from build123d import *

# Parameters (mm, degrees)
F1_DEPTH = 76.2
F2_R     = 46.767549
F3_DEPTH = 50.8


with BuildPart() as f1:
    # F0 (on Right) → F1 (new body)
    with BuildSketch(Plane.YZ):
        with BuildLine():
            ThreePointArc((-47.755212, -55.394912), (-16.585087, -35.145607), (-4.485609, 0))
            ThreePointArc((-4.485609, 0), (-16.585087, 35.145607), (-47.755212, 55.394912))
            ThreePointArc((-47.755212, 55.394912), (-118.673271, 0), (-47.755212, -55.394912))
        make_face()
        with BuildLine():
            ThreePointArc((-47.755212, 55.394912), (-16.585087, 35.145607), (-4.485609, 0))
            ThreePointArc((-4.485609, 0), (-16.585087, -35.145607), (-47.755212, -55.394912))
            Line((-47.755212, -55.394912), (75.465698, -24.644182))
            ThreePointArc((75.465698, -24.644182), (43.915552, 0), (75.465698, 24.644182))
            Line((75.465698, 24.644182), (-47.755212, 55.394912))
        make_face()
        with BuildLine():
            ThreePointArc((94.715552, 0), (89.332716, 15.635637), (75.465698, 24.644182))
            ThreePointArc((75.465698, 24.644182), (43.915552, 0), (75.465698, -24.644182))
            ThreePointArc((75.465698, -24.644182), (89.332716, -15.635637), (94.715552, 0))
        make_face()
    extrude(amount=F1_DEPTH)

    # F2 (on face) → F3 (cut)
    with BuildSketch(Plane.YZ.offset(76.2)):
        with Locations((-61.57944, 0)):
            Circle(F2_R)
    extrude(amount=-F3_DEPTH, mode=Mode.SUBTRACT)


solid = f1.part
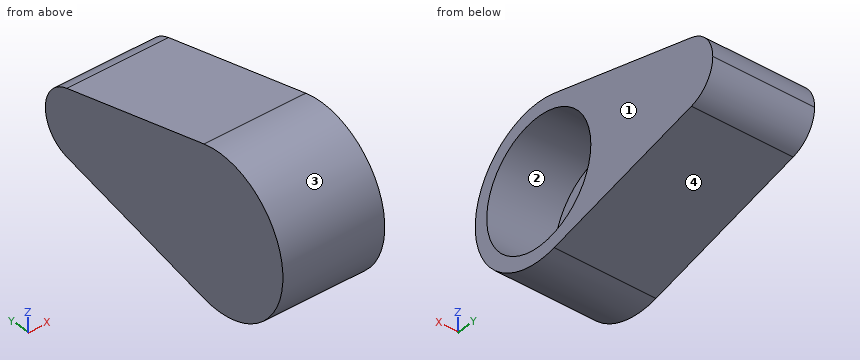
CAD build for the part. Positions are in the model's coordinates, mm. Face numbers are marked on the shaded views. Give positions to 0.01 mm unless a question says otherwise; leave off trailing zeros. Write each loop counter-clockwise with the first axis right and the second up, starting at its lowest first coordinate (ties: lowest second). Pieces come first, ordered by that corner, then holes. Notation, with made-up numbers: (37, -30.75) - (92, -30.75) arc R16 ccw to (92, -13.75) - close; hole circle Ø8 at (88.25, 52). An arc over 180 degrees is marked (long way). Put each result on its own line as item: value.
(1) Pull direction Y, two halves, no side cores. Call the marked faces 1, 2, 3 and 4: released by +Y, released by -Y, zero draft, split by the parting line, or undercut.
Working result:
face 1: zero draft
face 2: undercut
face 3: split by the parting line
face 4: released by +Y
(2) Saw through at B-B (z = -42.5). List the corners of the cut face in (x, y).
Working result:
outline: (0, -99.7) - (76.2, -99.7) - (76.2, -81.1) - (25.4, -81.1) - (25.4, -42.06) - (76.2, -42.06) - (76.2, 3.92) - (0, 3.92) - close
(3) Wall check: L1, parallel to X at y = -64, z = 41; L2, parallel to Z at x = 58, y = -30; L3, parallel to Z at x = 59, y = -70.5. Give the ranges that are in metal, low to high.
Working result:
L1: 0 to 25.4
L2: -50.96 to -34.5, 34.5 to 50.96
L3: -56.39 to -45.91, 45.91 to 56.39
(4) Saw through at C-C (y = -79). List the corners of the cut face in (x, z).
Working result:
outline: (0, -54.37) - (76.2, -54.37) - (76.2, -43.4) - (25.4, -43.4) - (25.4, 43.4) - (76.2, 43.4) - (76.2, 54.37) - (0, 54.37) - close
(5) Drop flat-ended pins along their axis: pin 1 Ø5 at (x, y) = (37, -36.5) entering from -Z; pin 2 Ø2 at (x, y) = (66, 13.5) entering from -Z; pin 3 Ø5 at (x, z) = (52.5, 35.5) entering from -Y. Give the stop position or say it passes through.
Working result:
pin 1: z = -53.21
pin 2: z = -40.36
pin 3: y = -108.17
(6) Saw through at D-D (x = 10.5). List the corners of the cut face in (y, z).
Working result:
outline: (-47.76, -55.39) - (75.47, -24.64) arc R25.4 ccw to (75.47, 24.64) - (-47.76, 55.39) arc R57.09 ccw (long way) to start
(7) Saw through at A-A (x = 33). List the corners of the cut face in (y, z), then the cut area to 3 significant figures.
Working result:
outline: (-47.76, -55.39) - (75.47, -24.64) arc R25.4 ccw to (75.47, 24.64) - (-47.76, 55.39) arc R57.09 ccw (long way) to start; hole circle Ø93.54 at (-61.58, 0)
area: 10,400 mm^2
